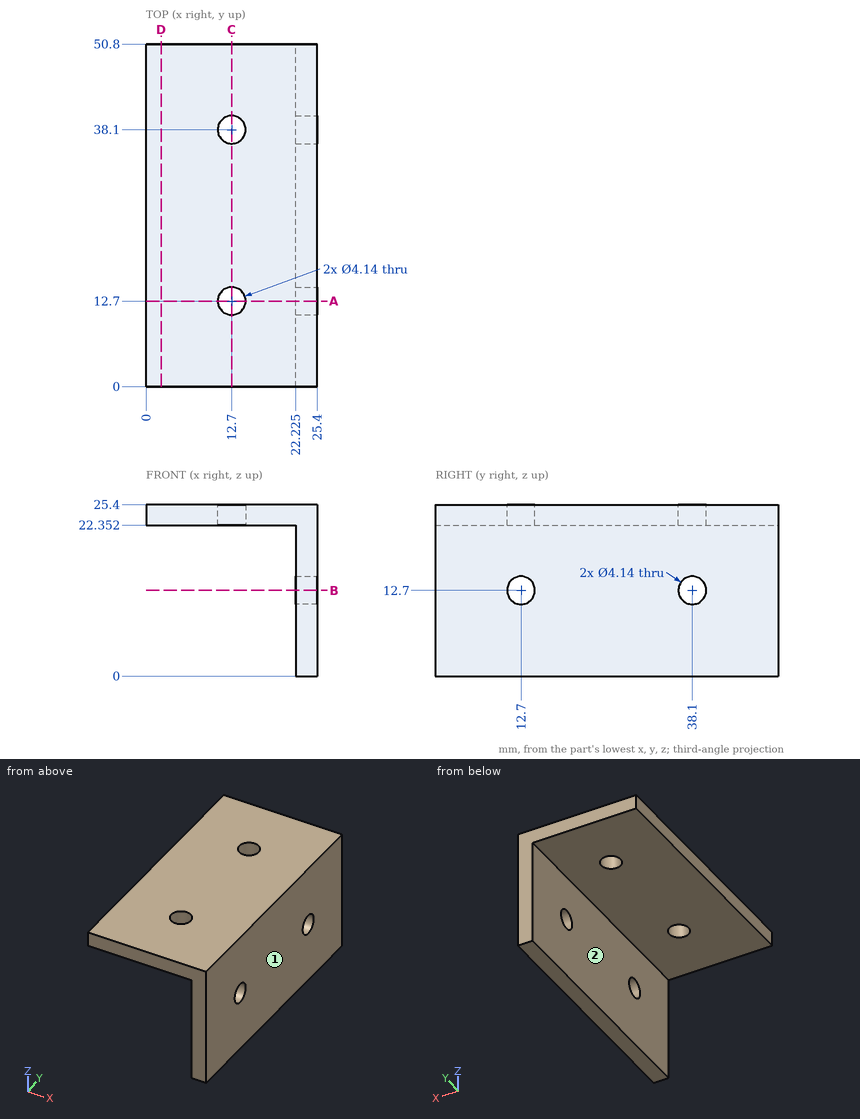
Answer from the drawing. Dimensions are ordinates in mm from the lowest x, y and z of the part. A direction names the side the tool comes from. Round coordinates to 2 decimals unless told otherwise and drop trailing zeros. Write each loop counter-clockwise with the first axis right and the second up, starting at its lowest first coordinate (ties: lowest second). Pieces come first, ordered by that corner, then holes. Notation, with made-up numbers: (76, 0.25) -> (114, 0.25) arc R7 cw to (114, 12.25) -> close; hole circle Ø3 at (38, 33.5). An arc over 180 degrees is marked (long way). Answer in a Markdown table with one row per item. Add a question column.
1) Which of the six approach directions +Z, -Z, +X, -X, +Y, -Y give full straight-line access (tool end or side, diameter ignored) to the marked faces 1 and 2?
2) Find section B-B, the plane z = 12.7. Determine the outline of the cut face in (x, y) (1 decimal), and give its area (3 significant figures).
3) Given P1, Ø6.5, axis at x = 16, y = 17, coming from the -Z side; P2, Ø4, axis at x = 9, z = 20, coming from the +Y side; P3, Ø10, axis at y = 36.5, z = 7, coming from the -X side (3 decimals), each flat-ended and moving along its own axis, determine where each tip first touches the part or whether it passes through.
4) Find section C-C, the plane x = 12.7. Determine the outline of the cut face in (y, z).
5) Consider line 1 (Y direction, x = 12.7, z = 24.6); line 2 (Z direction, x = 21, y = 5.5); line 3 (X direction, y = 6, z = 10.5) (3 decimals). Determine where each line is inside the solid, lowest interval first.
6) Find section A-A, the plane y = 12.7. Determine the outline of the cut face in (x, z) (1 decimal), and give its area (3 significant figures).
7) Find section D-D, the plane x = 2.25. Determine the outline of the cut face in (y, z).
Findings below:
| question | item | result |
|---|---|---|
| 1 | face 1 | +Z, -Z, +X, +Y, -Y |
| 1 | face 2 | -Z, -X, +Y, -Y |
| 2 | outline | (22.2, 0) -> (25.4, 0) -> (25.4, 10.6) -> (22.2, 10.6) -> close; (22.2, 14.8) -> (25.4, 14.8) -> (25.4, 36) -> (22.2, 36) -> close; (22.2, 40.2) -> (25.4, 40.2) -> (25.4, 50.8) -> (22.2, 50.8) -> close |
| 2 | area | 135 mm² |
| 3 | P1 | z = 22.35 |
| 3 | P2 | through |
| 3 | P3 | x = 22.225 |
| 4 | outline | (0, 22.35) -> (10.63, 22.35) -> (10.63, 25.4) -> (0, 25.4) -> close; (14.77, 22.35) -> (36.03, 22.35) -> (36.03, 25.4) -> (14.77, 25.4) -> close; (40.17, 22.35) -> (50.8, 22.35) -> (50.8, 25.4) -> (40.17, 25.4) -> close |
| 5 | line 1 | 0 to 10.63, 14.77 to 36.03, 40.17 to 50.8 |
| 5 | line 2 | 22.35 to 25.4 |
| 5 | line 3 | 22.225 to 25.4 |
| 6 | outline | (0, 22.4) -> (10.6, 22.4) -> (10.6, 25.4) -> (0, 25.4) -> close; (14.8, 22.4) -> (22.2, 22.4) -> (22.2, 14.8) -> (25.4, 14.8) -> (25.4, 25.4) -> (14.8, 25.4) -> close; (22.2, 0) -> (25.4, 0) -> (25.4, 10.6) -> (22.2, 10.6) -> close |
| 6 | area | 123 mm² |
| 7 | outline | (0, 22.35) -> (50.8, 22.35) -> (50.8, 25.4) -> (0, 25.4) -> close |
